For this review, take the finished solid that the model builds, in its own axes (mm). Give positions to 0.01 mm unless a question says otherwise; leave off trailing zeros. Loops run counter-clockwise (first coordinate to the right, second up) from the corner with the lowest first, then second, coordinate; pieces in that order, holes last. Notation, with made-up numbers: (30, 2.25) -> (71, 2.25) arc R25 cw to (71, 15.25) -> close; hole circle Ø10 at (-28, -37.5). An arc over 180 degrees is marked (long way). Answer as CSV lines item,"result". Start each with the question number.
Item 1: For L1, parallel to Y at x = 0, z = 1.9; L2, parallel to X at y = 13, z = 3.5; L3, parallel to Y at x = 1, z = 1.2, list the stretches that pass through material, from the lowest coordinate up. Write a range as from..to.
Item 2: Add section D-D on x = 4. State the section outline as (y, z) points.
Item 3: Clearance check with flat-ended pins moving along their axes: P1, Ø4, axis at x = 0, y = -35, coming from the +Z side; P2, Ø2, axis at x = -1.5, z = 2.5, coming from the -Y side. State where each tip first meets the part, or that it passes through.
Item 4: Add section A-A on x = 0. State the section outline as (y, z) points.
Item 5: Add section B-B on y = -2.5. State the section outline as (x, z) points, plus the area to 3 significant figures.
Item 6: Add section C-C on z = 2.75. State the section outline as (x, y) points.
Autodesk Inventor part; units mm, degrees
ref_plane "YZ Plane" through (0, 0, 0) normal (1, 0, 0) x (0, 1, 0)
ref_plane "XZ Plane" through (0, 0, 0) normal (0, 1, 0) x (-1, 0, 0)
ref_plane "XY Plane" through (0, 0, 0) normal (0, 0, 1) x (1, 0, 0)
sketch "Эскиз1" plane through (0, 0, 0) normal (0, 0, 1) x (1, 0, 0)
  arc A0 (5, 35) -> (-5, 35) centre (0, 35) ccw
  line L0 (-5, 35) -> (-5, -35)
  arc A1 (-5, -35) -> (5, -35) centre (0, -35) ccw
  line L1 (5, -35) -> (5, 35)
  arc A2 (-1.6, -30.2629) -> (1.6, -30.2629) centre (0, -30.2629) ccw
  line L2 (-1.6, -30.2629) -> (-1.6, 35)
  arc A3 (1.6, 35) -> (-1.6, 35) centre (0, 35) ccw
  line L3 (1.6, 35) -> (1.6, -30.2629)
  circle A4 centre (0, -35) radius 1.6
  point P0 (0, 0)
extrude "Выдавливание1" add sketch "Эскиз1" along normal blind 4
properties part number "holder"
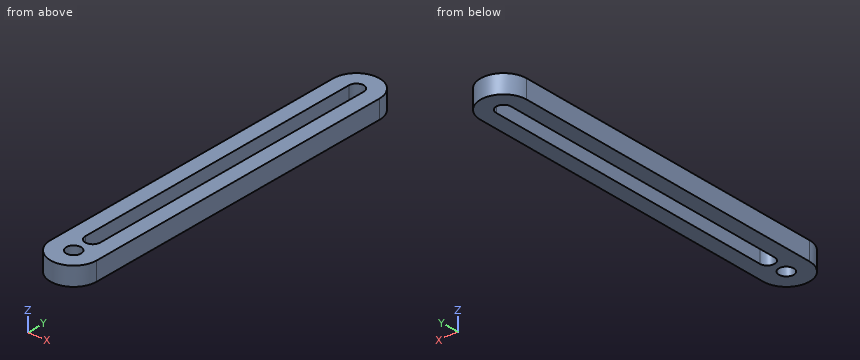
Computed values:
1,L1,"-40..-36.6, -33.4..-31.86, 36.6..40"
1,L2,"-5..-1.6, 1.6..5"
1,L3,"-39.9..-36.25, -33.75..-31.51, 36.25..39.9"
2,outline,"(-38, 0) -> (38, 0) -> (38, 4) -> (-38, 4) -> close"
3,P1,"z = 4"
3,P2,"y = -39.97"
4,outline,"(-40, 0) -> (-36.6, 0) -> (-36.6, 4) -> (-40, 4) -> close; (-33.4, 0) -> (-31.86, 0) -> (-31.86, 4) -> (-33.4, 4) -> close; (36.6, 0) -> (40, 0) -> (40, 4) -> (36.6, 4) -> close"
5,outline,"(-5, 0) -> (-1.6, 0) -> (-1.6, 4) -> (-5, 4) -> close; (1.6, 0) -> (5, 0) -> (5, 4) -> (1.6, 4) -> close"
5,area,"27.2 mm²"
6,outline,"(-5, -35) arc R5 ccw to (5, -35) -> (5, 35) arc R5 ccw to (-5, 35) -> close; hole circle Ø3.2 at (0, -35); hole (-1.6, -30.26) arc R1.6 ccw to (1.6, -30.26) -> (1.6, 35) arc R1.6 ccw to (-1.6, 35) -> close"
